Design review of the part shown in the three views and the two pictorial views. Dimensions are in mm from the part's minimum x, y and z. A direction names the side the tool comes from. Coordinates: 2 decimals unless noted, no trailing zeros. Write each loop counter-clockwise with the first axis right and the second up, starting at its lowest first coordinate (ties: lowest second). Pieces come first, ordered by that corner, then holes.
Q1. For pin 1 Ø12.5 at (y, z) = (37.5, 10.5) entering from +X (1 decimal); pin 2 Ø20 at (x, y) = (50.5, 29.5) entering from -Z; pin 3 Ø8 at (x, y) = (32, 8.5) entering from -Z, all flat-tipped, find the tip position at first contact; note any pin that passes through.
Q2. The part is to be moulded in two halves that separate along X. For the marked faces 1, 2 and 3, say which applies: released by +X, released by -X, zero draft, split by the parting line, or undercut.
Q3. For the marked faces 4, 5 and 6, list the 3-axis set-ups (+Z, -Z, +X, -X, +Y, -Y) from which the entire face can be reached by the end or side of a thin tool; tool diameter is ignored.
Q4. For L1, parallel to X at y = 34.5, z = 10 (1 decimal); L2, parallel to Y at x = 22, z = 25 (1 decimal); L3, parallel to Y at x = 43, z = 15.5 (1 decimal), list the stretches that pass through material, from the lowest coordinate up.
Q5. Take a section at C-C, the plane z = 10. Write out the cut boundary in (x, y) (1 decimal), plus the area to 3 significant figures.
Q6. Take a section at B-B, the plane z = 24. Write out the cut boundary in (x, y) (1 decimal).
Q7. Take a section at D-D, the plane y = 34. Write out the cut boundary in (x, z) (1 decimal), plus the area to 3 significant figures.
Q8. Take a section at A-A, the plane y = 8.5. Write out the cut boundary in (x, z) (1 decimal), plus the area to 3 significant figures.
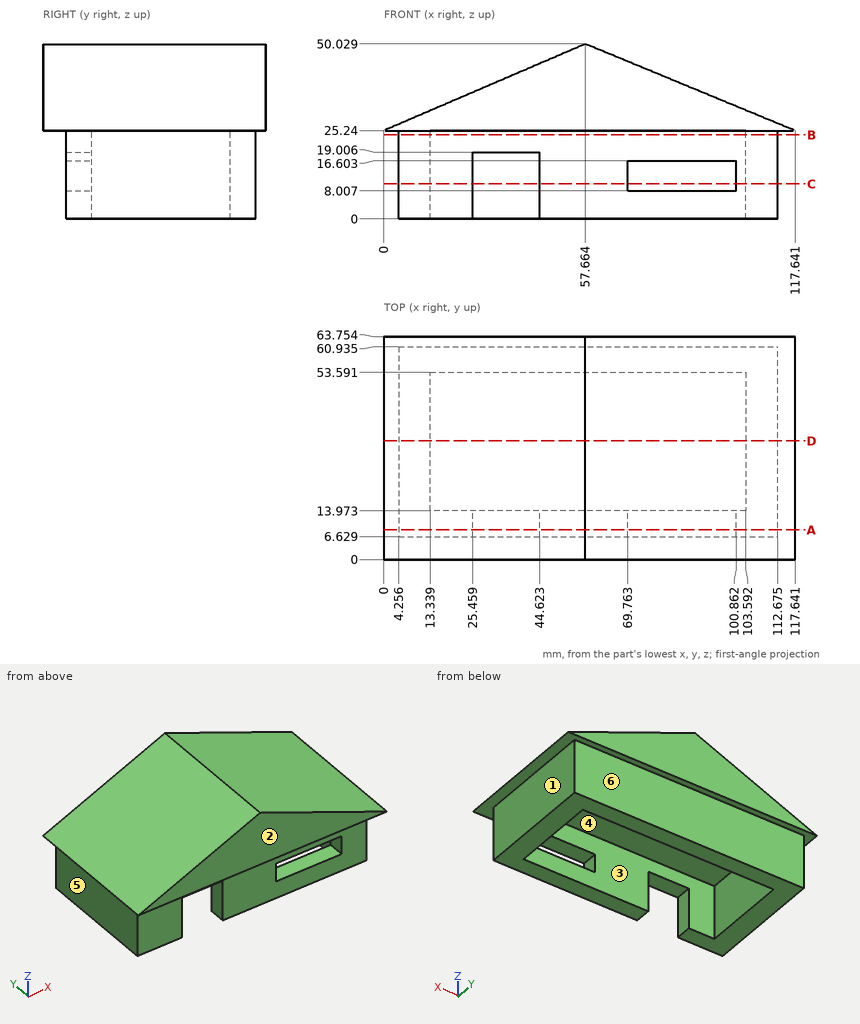
Responses:
1. pin 1: stops at x = 112.7
1. pin 2: stops at z = 25.24
1. pin 3: stops at z = 19.01
2. face 1: released by +X
2. face 2: zero draft
2. face 3: undercut
3. face 4: -Z
3. face 5: -Z, -X, +Y, -Y
3. face 6: -Z, +X, -X, +Y
4. L1: x = 4.3 to 13.3, 103.6 to 112.7
4. L2: y = 6.6 to 14, 53.6 to 60.9
4. L3: y = 53.6 to 60.9
5. outline: (4.3, 6.6) - (25.5, 6.6) - (25.5, 14) - (13.3, 14) - (13.3, 53.6) - (103.6, 53.6) - (103.6, 14) - (100.9, 14) - (100.9, 6.6) - (112.7, 6.6) - (112.7, 60.9) - (4.3, 60.9) - close; (44.6, 6.6) - (69.8, 6.6) - (69.8, 14) - (44.6, 14) - close
5. area: 1,940 mm2
6. outline: (4.3, 6.6) - (112.7, 6.6) - (112.7, 60.9) - (4.3, 60.9) - close; hole (13.3, 14) - (103.6, 14) - (103.6, 53.6) - (13.3, 53.6) - close
7. outline: (0, 25.2) - (4.3, 25.2) - (4.3, 0) - (13.3, 0) - (13.3, 25.2) - (103.6, 25.2) - (103.6, 0) - (112.7, 0) - (112.7, 25.2) - (117.6, 25.2) - (57.7, 50) - close
7. area: 1,920 mm2
8. outline: (0, 25.2) - (4.3, 25.2) - (4.3, 0) - (25.5, 0) - (25.5, 19) - (44.6, 19) - (44.6, 0) - (112.7, 0) - (112.7, 25.2) - (117.6, 25.2) - (57.7, 50) - close; hole (69.8, 8) - (100.9, 8) - (100.9, 16.6) - (69.8, 16.6) - close
8. area: 3,560 mm2
